The model under review builds one solid part; all positions refer to its coordinate system, in mm. Give positions to 0.01 mm unless a question says otherwise; leave off trailing zeros. Order: outer loops, then holes, each group sorted by start corner. A loop starts at its lowest first (then second) coordinate and runs counter-clockwise, first axis right, second up.
```python
from build123d import *

# Parameters (mm, degrees)
SKETCH1_W           = 25.4
SKETCH1_H           = 38.1
SKETCH1_W_2         = 12.7
SKETCH1_H_2         = 12.7
BOSS_EXTRUDE1_DEPTH = 3.175
SKETCH2_R           = 2.032
BOSS_EXTRUDE2_DEPTH = 3.175
SKETCH2_3_R         = 3.95
CUT_EXTRUDE1_DEPTH  = 63.201892938
FILLET1_R           = 2.54


with BuildPart() as part:
    # Sketch1 → Boss-Extrude1 (new body)
    with BuildSketch(Plane(origin=(0, 0, 0), x_dir=(1, 0, 0), z_dir=(0, 1, 0))):
        Rectangle(SKETCH1_W, SKETCH1_H)
        with Locations((19.05, -12.7)):
            Rectangle(SKETCH1_W_2, SKETCH1_H_2)
    extrude(amount=BOSS_EXTRUDE1_DEPTH)

    # Sketch2 → Boss-Extrude2 (add)
    # profile 1 of 2: a face of its own
    with BuildSketch(Plane.XZ):
        Polygon((12.7, 1.472649747), (13.949167892, 4.789594929), (12.7, 5.186439946), align=None)
    # profile 2 of 2: a face of its own
    with BuildSketch(Plane.XZ):
        with BuildLine():
            Line((-12.7, 13.255702289), (-13.373056837, 13.469524029))
            ThreePointArc((-13.373056837, 13.469524029), (-13.831582673, 13.569694165), (-14.300710901, 13.583790422))
            ThreePointArc((-14.300710901, 13.583790422), (-16.90590193, 12.668940106), (-18.647730427, 10.526510437))
            Line((-18.647730427, 10.526510437), (-33.997782473, -25.04377908))
            ThreePointArc((-33.997782473, -25.04377908), (-34.900150323, -28.214966504), (-34.955795775, -31.511570969))
            Line((-34.955795775, -31.511570969), (-34.123437377, -38.826910048))
            ThreePointArc((-34.123437377, -38.826910048), (-32.117046877, -43.516551498), (-27.863250656, -46.331432931))
            Line((-27.863250656, -46.331432931), (-12.15852304, -51.079668538))
            ThreePointArc((-12.15852304, -51.079668538), (-8.439878849, -50.772366449), (-5.934296975, -48.007441738))
            Line((-5.934296975, -48.007441738), (-0.611549336, -33.873823471))
            Line((-0.611549336, -33.873823471), (4.971130901, -19.05))
            Line((4.971130901, -19.05), (-12.7, -19.05))
            Line((-12.7, -19.05), (-12.7, 8.957831881))
            Line((-12.7, 8.957831881), (-12.7, 13.255702289))
        make_face()
        with Locations(Location((-7.764936406, -34.507055205, 0), (0, 0, 270))):
            Circle(SKETCH2_R, mode=Mode.SUBTRACT)
        with Locations(Location((-27.434824274, -26.25669415, 0), (0, 0, 270))):
            Circle(SKETCH2_R, mode=Mode.SUBTRACT)
    extrude(amount=-BOSS_EXTRUDE2_DEPTH)

    # Sketch2_3 → Cut-Extrude1 (cut, through all)
    with BuildSketch(Plane.XZ):
        Polygon((-12.7, 13.255702289), (12.7, 5.186439946), (12.7, 6.35), (25.4, 6.35), (25.4, 19.05), (-12.7, 19.05), align=None)
        Polygon((12.7, -19.05), (12.7, 1.472649747), (4.971130901, -19.05), align=None)
        with Locations(Location((-2.723911437, -9.485123164, 0), (0, 0, 270))):
            Circle(SKETCH2_3_R)
    extrude(amount=-CUT_EXTRUDE1_DEPTH, mode=Mode.SUBTRACT)

    # Fillet1
    fillet1_edges = [part.edges().sort_by_distance(p)[0] for p in [
        (13.949167892, 1.5875, 4.789594929),
    ]]
    fillet(fillet1_edges, radius=FILLET1_R)


solid = part.part
```
Item 1: Draft analysis for pull direction X (two halves, no side actions). For faces 1 (the cylindrical face through (-7.676, 1.565, -32.477)), 2 (the cylindrical face through (-16.874, 1.565, 12.691)), 3 (the flat face through (-11, 3.175, -18)), 4 (the cylindrical face through (-8.5, 1.6, -50.8)), state which applies: released by +X, released by -X, zero draft, split by the parting line, or undercut.
Values found:
face 1: undercut
face 2: released by -X
face 3: zero draft
face 4: split by the parting line
Item 2: For line 1 (Z direction, x = -9, y = 0.85); line 2 (Z direction, x = -27.5, y = 1.9); line 3 (X direction, y = 1.1, z = -35.5), list the stretches that pass through material, from the lowest coordinate up.
Values found:
line 1: z = -51.01 to -36.12, -32.89 to 12.08
line 2: z = -46.44 to -28.29, -24.23 to -9.99
line 3: x = -34.5 to -9.54, -5.99 to -1.22
Item 3: Take a section at D-D (z = -47). Give the boundary of the cut face in (x, y) (3 decimals).
Values found:
outline: (-25.652, 0) - (-5.555, 0) - (-5.555, 3.175) - (-25.652, 3.175) - close
Item 4: Clearance check with flat-ended pins moving along their axes: pin 1 Ø1.5 at (y, z) = (0.5, -35) entering from +X; pin 2 Ø1 at (y, z) = (2, -33.5) entering from -X. State where each tip first meets the part, or that it passes through.
Values found:
pin 1: stops at x = -0.75
pin 2: stops at x = -34.79
Item 5: Take a section at C-C (y = 2.35). Give the number of separate pieces and of enclosed holes in the cut face, and give its area (3 significant figures).
Values found:
separate pieces: 1
enclosed holes: 3
area: 1,920 mm2
Item 6: Take a section at B-B (x = -22.5). Give the boundary of the cut face in (y, z) (3 decimals), and give its area (3 significant figures).
Values found:
outline: (0, -47.953) - (3.175, -47.953) - (3.175, 1.6) - (0, 1.6) - close
area: 157 mm2
Item 7: Take a section at A-A (x = -8.5). Give the boundary of the cut face in (y, z) (3 decimals), and give its area (3 significant figures).
Values found:
outline: (0, -50.802) - (3.175, -50.802) - (3.175, -36.401) - (0, -36.401) - close; (0, -32.613) - (3.175, -32.613) - (3.175, 11.921) - (0, 11.921) - close
area: 187 mm2
